Read the model definition and answer for the solid it produces. Units are mm, in the model's axes. A direction names the side the tool comes from. Coordinates: 2 decimals unless noted, no trailing zeros. Write each loop counter-clockwise with the first axis right and the second up, starting at its lowest first coordinate (ties: lowest second). Pieces come first, ordered by that corner, then holes. Notation, with made-up numbers: (63, 47.25) -> (98, 47.25) arc R13 cw to (98, 60.25) -> close; hole circle Ø1 at (38, 59.25). An arc over 180 degrees is marked (long way). Use CSV: the item, a comma, the result in double quotes.
Autodesk Inventor part; units mm, degrees
ref_plane "YZ Plane" through (0, 0, 0) normal (1, 0, 0) x (0, 1, 0)
ref_plane "XZ Plane" through (0, 0, 0) normal (0, 1, 0) x (-1, 0, 0)
ref_plane "XY Plane" through (0, 0, 0) normal (0, 0, 1) x (1, 0, 0)
ref_plane "Work Plane1" through (0, 0, 0) normal (0, 0, 1) x (1, 0, 0)
sketch "Sketch1" plane through (0, 0, 0) normal (0, 0, 1) x (1, 0, 0)
  line L0 (-32.75, 0) -> (32.75, 0)
  arc A0 (37.75, -5) -> (32.75, 0) centre (32.75, -5) ccw
  line L1 (37.75, -5) -> (37.75, -15)
  line L2 (-37.75, -20) -> (77.75, -20) construction
  line L3 (0.95, -48) -> (37.75, -48) construction
  arc A1 (32.75, -68) -> (37.75, -63) centre (32.75, -63) ccw
  line L4 (37.75, -63) -> (37.75, -48)
  line L5 (26.6, -68) -> (32.75, -68)
  line L6 (19.75, 0) -> (37.75, 0)
  line L7 (37.75, 0) -> (37.75, -68)
  line L8 (37.75, -68) -> (19.75, -68)
  line L9 (19.75, -68) -> (19.75, 0)
  point P0 (0, 0)
  point P1 (24.75, -5)
  point P2 (24.75, -63)
  dimension "d0" = 18
  dimension "d1" = 5
  dimension "d2" = 5
  dimension "d3" = 5
extrude "Extrusion1" add sketch "Sketch1" along normal blind 7 contours L0 A0 L1 L7 L4 A1 L5 L8 L9
sketch "Sketch2" plane through (0, 0, 0) normal (0, 0, -1) x (-1, 0, 0)
  line L0 (37.75, -20) -> (-77.75, -20) construction
  line L1 (-0.95, -48) -> (-37.75, -48)
  line L2 (-19.75, 0) -> (-19.75, -68)
  line L3 (-37.75, -63) -> (-37.75, -5)
  line L4 (-19.75, -48) -> (-37.75, -48)
  line L5 (-37.75, -48) -> (-37.75, -20)
  line L6 (-37.75, -20) -> (-19.75, -20)
  line L7 (-19.75, -20) -> (-19.75, -48)
  point P0 (0, 0)
  point P1 (-19.75, -20)
extrude "Extrusion2" cut sketch "Sketch2" against normal blind 2
sketch "Sketch3" plane through (0, 0, 7) normal (0, 0, 1) x (1, 0, 0)
  line L0 (19.75, -68) -> (32.75, -68)
  arc A0 (32.75, -68) -> (37.75, -63) centre (32.75, -63) ccw
  line L1 (37.75, -63) -> (37.75, -5)
  arc A1 (37.75, -5) -> (32.75, 0) centre (32.75, -5) ccw
  line L2 (32.75, 0) -> (19.75, 0)
  line L3 (19.75, 0) -> (19.75, -68)
  line L4 (37.75, -34) -> (19.75, -34) construction
  line L5 (28.75, -34) -> (28.75, -68) construction
  line L6 (19.75, -68) -> (32.75, -68)
  line L7 (-37.75, -20) -> (77.75, -20) construction
  line L8 (0.95, -48) -> (37.75, -48)
  line L9 (77.75, -15) -> (37.75, -15)
  point P0 (0, 0)
  point P1 (32.75, -63)
  point P2 (32.75, -15)
  point P3 (32.75, -53)
  point P4 (24.75, -15)
  point P5 (24.75, -53)
  dimension "d15" = 5
  dimension "d16" = 5
  dimension "d22" = 5
  dimension "d23" = 5
hole "Hole1" at (32.75, -5, 7) at (32.75, -63, 7) at (32.75, -15, 7) at (24.75, -15, 7) at (24.75, -53, 7) at (32.75, -53, 7) direction (0, 0, -1) diameter 3.4 depth 7 counterbore diameter 6.5 counterbore depth 3.4
chamfer "Chamfer1" distance 12 angle 45 2 edges at (19.75, -68, 3.5) (19.75, 0, 3.5)
properties part number "SideBrace"
1. Each of these flat-tipped pins is pushed along its axis until it touches: pin 1 Ø1 at (x, y) = (23.5, -40.5) entering from -Z; pin 2 Ø2 at (x, z) = (29.5, 4) entering from +Y; pin 3 Ø3 at (x, y) = (25.5, -52.5) entering from +Z. Where does it stop, or does it pass through?
Solutions:
pin 1,"stops at z = 2"
pin 2,"stops at y = -1.25"
pin 3,"stops at z = 3.6"
2. A tool of negligible diameter and unlimited length cuts with its end or side. For faces 1 (the cylindrical face through (34.26, -15.78, 1.77)), 2 (the cylindrical face through (27.923, -14.295, 5.276)), 3 (the flat face through (29, -20, 1)), from which of +Z, -Z, +X, -X, +Y, -Y can it reach the whole face along a straight path? Write none if from no direction.
Solutions:
face 1,"+Z, -Z"
face 2,"+Z"
face 3,"-Z, +X, -X"
3. Find the intervals of material crossed by line 1 along Y through (x, z) = (32.75, 5.85); line 2 along X through (y, z) = (-53, 6.3); line 3 along Y through (x, z) = (32.75, 1.55), in increasing order.
Solutions:
line 1,"y = -68 to -66.25, -59.75 to -56.25, -49.75 to -18.25, -11.75 to -8.25, -1.75 to 0"
line 2,"x = 19.75 to 21.5, 28 to 29.5, 36 to 37.75"
line 3,"y = -68 to -64.7, -61.3 to -54.7, -51.3 to -48, -20 to -16.7, -13.3 to -6.7, -3.3 to 0"
4. A cutting plane is placed at C-C (y = -15). Give the vertices of the cut face in (x, z).
Solutions:
outline,"(19.75, 0) -> (23.05, 0) -> (23.05, 3.6) -> (21.5, 3.6) -> (21.5, 7) -> (19.75, 7) -> close; (26.45, 0) -> (31.05, 0) -> (31.05, 3.6) -> (29.5, 3.6) -> (29.5, 7) -> (28, 7) -> (28, 3.6) -> (26.45, 3.6) -> close; (34.45, 0) -> (37.75, 0) -> (37.75, 7) -> (36, 7) -> (36, 3.6) -> (34.45, 3.6) -> close"
5. A cutting plane is placed at A-A (z = 1.25). Give the vertices of the cut face in (x, y).
Solutions:
outline,"(19.75, -56) -> (31.75, -68) -> (32.75, -68) arc R5 ccw to (37.75, -63) -> (37.75, -48) -> (19.75, -48) -> close; (19.75, -20) -> (37.75, -20) -> (37.75, -5) arc R5 ccw to (32.75, 0) -> (31.75, 0) -> (19.75, -12) -> close; hole circle Ø3.4 at (24.75, -53); hole circle Ø3.4 at (24.75, -15); hole circle Ø3.4 at (32.75, -63); hole circle Ø3.4 at (32.75, -53); hole circle Ø3.4 at (32.75, -15); hole circle Ø3.4 at (32.75, -5)"
6. For a pull along X with two mould halves and no side action, classify faces 4 (the flat face through (29, -34, 2)), 5 (the flat face through (26.1, -16.4, 3.6)), 6 (the flat face through (19.75, -34, 4)), 7 (the cylindrical face through (36.25, -1.43, 3.45)) as pulls with the +X half, pulls with the -X half, needs draft (parallel to the pull), parting line crosses it, or undercut.
Solutions:
face 4,"needs draft"
face 5,"undercut"
face 6,"pulls with the -X half"
face 7,"pulls with the +X half"
7. A cutting plane is placed at B-B (x = 24.75). Give the vertices of the cut face in (y, z).
Solutions:
outline,"(-61, 0) -> (-54.7, 0) -> (-54.7, 3.6) -> (-56.25, 3.6) -> (-56.25, 7) -> (-61, 7) -> close; (-51.3, 0) -> (-48, 0) -> (-48, 2) -> (-20, 2) -> (-20, 0) -> (-16.7, 0) -> (-16.7, 3.6) -> (-18.25, 3.6) -> (-18.25, 7) -> (-49.75, 7) -> (-49.75, 3.6) -> (-51.3, 3.6) -> close; (-13.3, 0) -> (-7, 0) -> (-7, 7) -> (-11.75, 7) -> (-11.75, 3.6) -> (-13.3, 3.6) -> close"
8. A cutting plane is placed at D-D (y = -58). Give the vertices of the cut face in (x, z), and give its area (3 significant figures).
Solutions:
outline,"(21.75, 0) -> (37.75, 0) -> (37.75, 7) -> (21.75, 7) -> close"
area,"112 mm^2"
